from build123d import *

# Parameters (mm, degrees)
SKETCH1_W           = 38.200952294
SKETCH1_H           = 25.337366318
BOSS_EXTRUDE1_DEPTH = 1.6764
SKETCH2_R           = 1.524
CUT_EXTRUDE1_DEPTH  = 1.6764
SKETCH5_W           = 7.761339033
SKETCH5_H           = 5.842
BOSS_EXTRUDE2_DEPTH = 7.62


with BuildPart() as part:
    # Sketch1 → Boss-Extrude1 (new body)
    with BuildSketch(Plane(origin=(0, 0, 0), x_dir=(1, 0, 0), z_dir=(0, 1, 0))):
        Rectangle(SKETCH1_W, SKETCH1_H)
    extrude(amount=BOSS_EXTRUDE1_DEPTH)

    # Sketch2 → Cut-Extrude1 (cut)
    with BuildSketch(Plane(origin=(0, 1.6764, 0), x_dir=(1, 0, 0), z_dir=(0, 1, 0))):
        with Locations(Location((-15.849276147, -9.404783159, 0), (0, 0, 270))):
            Circle(SKETCH2_R)
        with Locations(Location((-15.849276147, 9.493683159, 0), (0, 0, 270))):
            Circle(SKETCH2_R)
        with Locations(Location((15.912776147, 9.519083159, 0), (0, 0, 270))):
            Circle(SKETCH2_R)
        with Locations(Location((15.900076147, -9.468283159, 0), (0, 0, 270))):
            Circle(SKETCH2_R)
    extrude(amount=-CUT_EXTRUDE1_DEPTH, mode=Mode.SUBTRACT)

    # Sketch5 → Boss-Extrude2 (add)
    with BuildSketch(Plane.XZ):
        with Locations((15.219806631, -0.36511235)):
            Rectangle(SKETCH5_W, SKETCH5_H)
    extrude(amount=BOSS_EXTRUDE2_DEPTH)


solid = part.part
The listing builds one solid part. Answer for the finished solid, in the listing's coordinates (mm). A direction names the side the tool comes from. Round coordinates to 2 decimals unless told otherwise and drop trailing zeros. Order: outer loops, then holes, each group sorted by start corner. A loop starts at its lowest first (then second) coordinate and runs counter-clockwise, first axis right, second up. Notation, with made-up numbers: (40.5, 19.25) -> (55.5, 19.25) arc R26 cw to (55.5, 33.25) -> close; hole circle Ø3 at (-28.5, -16.75). An arc over 180 degrees is marked (long way). Put each result on its own line as item: value.
Q1. Section A-A, the plane z = -10 is taken. Write down the section's boundary in (x, y), and give its area (3 significant figures).
Results list:
outline: (-19.1, 0) -> (-17.29, 0) -> (-17.29, 1.68) -> (-19.1, 1.68) -> close; (-14.41, 0) -> (14.47, 0) -> (14.47, 1.68) -> (-14.41, 1.68) -> close; (17.36, 0) -> (19.1, 0) -> (19.1, 1.68) -> (17.36, 1.68) -> close
area: 54.4 mm^2
Q2. Which of the six approach directions +Z, -Z, +X, -X, +Y, -Y give full straight-line access (tool end or side, diameter ignored) to faces 1 (the flat face through (15, -7.62, 0)), 2 (the flat face through (15, -4, 2.556)), 3 (the flat face through (15, -4, -3.286))?
Results list:
face 1: +Z, -Z, +X, -X, -Y
face 2: +Z, +X, -X, -Y
face 3: -Z, +X, -X, -Y
Q3. Each of these flat-tipped pins is pushed along its axis until it touches: P1, Ø6, axis at x = -7.5, z = 7, coming from the -Y side; P2, Ø2.5, axis at x = -15.85, z = -9.49, coming from the -Y side; P3, Ø4.5, axis at y = -5, z = 0.5, coming from the -X side; P4, Ø2.5, axis at x = 14, y = -3.5, coming from the +Z side. Where does it stop, or does it pass through?
Results list:
P1: y = 0
P2: through
P3: x = 11.34
P4: z = 2.56
Q4. Section B-B, the plane x = 13.5 is taken. Write down the section's boundary in (y, z).
Results list:
outline: (-7.62, -3.29) -> (0, -3.29) -> (0, -12.67) -> (1.68, -12.67) -> (1.68, 12.67) -> (0, 12.67) -> (0, 2.56) -> (-7.62, 2.56) -> close
Q5. Section C-C, the plane y = 0.5 is taken. Write down the section's boundary in (x, z), and give its area (3 significant figures).
Results list:
outline: (-19.1, -12.67) -> (19.1, -12.67) -> (19.1, 12.67) -> (-19.1, 12.67) -> close; hole circle Ø3.05 at (-15.85, -9.49); hole circle Ø3.05 at (-15.85, 9.4); hole circle Ø3.05 at (15.9, 9.47); hole circle Ø3.05 at (15.91, -9.52)
area: 939 mm^2
Q6. Consider line 1 along Z through (x, y) = (16, 0.75); line 2 along Y through (x, z) = (-7.5, -2); line 3 along X through (y, z) = (-3, 0.75). Determine where each line is inside the solid, lowest interval first.
Results list:
line 1: -12.67 to -11.04, -8 to 7.95, 10.99 to 12.67
line 2: 0 to 1.68
line 3: 11.34 to 19.1
Q7. Determine the mould class of faces 4 (the cylindrical face through (14.425, 0.85, -9.849)), 5 (the flat face through (0, 1.676, 0)), 6 (the flat face through (11.339, -4, 0)) for opening direction X: pulls with the +X half, pulls with the -X half, needs draft (parallel to the pull), parting line crosses it, or undercut.
Results list:
face 4: undercut
face 5: needs draft
face 6: pulls with the -X half
Q8. Section D-D, the plane z = 5.5 is taken. Write down the section's boundary in (x, y).
Results list:
outline: (-19.1, 0) -> (19.1, 0) -> (19.1, 1.68) -> (-19.1, 1.68) -> close
